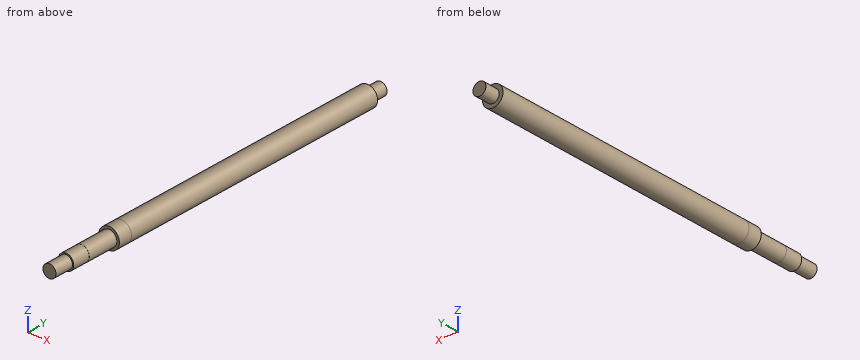
Autodesk Inventor part; units mm, degrees
ref_plane "YZ Plane" through (0, 0, 0) normal (1, 0, 0) x (0, 1, 0)
ref_plane "XZ Plane" through (0, 0, 0) normal (0, 1, 0) x (-1, 0, 0)
ref_plane "XY Plane" through (0, 0, 0) normal (0, 0, 1) x (1, 0, 0)
sketch "Sketch1" plane through (0, 0, 0) normal (0, 1, 0) x (-1, 0, 0)
  circle A0 centre (0, 0) radius 8
  dimension "d0" = 16
extrude "Extrusion1" add sketch "Sketch1" along normal blind 300
sketch "Sketch2" plane through (0, 0, 0) normal (0, -1, 0) x (1, 0, 0)
  circle A0 centre (0, 0) radius 8
extrude "Extrusion2" cut sketch "Sketch2" against normal blind 50
sketch "Sketch3" plane through (0, 50, 0) normal (0, -1, 0) x (1, 0, 0)
  circle A0 centre (0, 0) radius 8
extrude "Extrusion3" add sketch "Sketch3" along normal blind 50
sketch "Sketch4" plane through (0, 0, 0) normal (0, -1, 0) x (1, 0, 0)
  circle A0 centre (0, 0) radius 8
  circle A1 centre (0, 0) radius 6
  dimension "d7" = 12
extrude "Extrusion4" cut sketch "Sketch4" against normal blind 14
thread "Thread1"
sketch "Sketch6" plane through (0, 14, 0) normal (0, -1, 0) x (1, 0, 0)
  circle A0 centre (0, 0) radius 8
  circle A1 centre (0, 0) radius 6.05
  dimension "d13" = 12.1
extrude "Extrusion5" cut sketch "Sketch6" against normal blind 25
sketch "Sketch7" plane through (0, 0, 0) normal (0, -1, 0) x (1, 0, 0)
  circle A0 centre (0, 0) radius 6
  circle A1 centre (0, 0) radius 5
  dimension "d16" = 10
extrude "Extrusion6" add sketch "Sketch7" along normal blind 15 contours A1
sketch "Sketch8" plane through (0, 300, 0) normal (0, 1, 0) x (1, 0, 0)
  circle A0 centre (0, 0) radius 8
extrude "Extrusion7" cut sketch "Sketch8" against normal blind 27.101
sketch "Sketch9" plane through (0, 272.899, 0) normal (0, 1, 0) x (1, 0, 0)
  circle A0 centre (0, 0) radius 8
  circle A1 centre (0, 0) radius 5
  dimension "d21" = 10
extrude "Extrusion8" add sketch "Sketch9" along normal blind 12 contours A1
properties part number "1605_300mm"
Verification items for the finished model (mm, model axes). Coordinates: 2 decimals unless noted, no trailing zeros. Loops run counter-clockwise (first coordinate to the right, second up) from the corner with the lowest first, then second, coordinate; pieces in that order, holes last. Notation, with made-up numbers: (-24.75, -18) -> (-19.75, -18) arc R32 ccw to (-19.75, 8) -> close; hole circle Ø8 at (0.5, -29.75). An arc over 180 degrees is marked (long way). Answer as a JSON object with one key per item and string values. Group by question number.
Item 1: Sectioned sample at C-C on y = 123. Record the boundary of the cut face in (x, z), plus the area to 3 significant figures.
Item 2: Sectioned sample at B-B on x = 0. Record the boundary of the cut face in (y, z).
Item 3: Sectioned sample at A-A on z = 0. Record the boundary of the cut face in (x, y), plus the area to 3 significant figures.
Item 4: Scan lines: probe 1 along X at (y, z) = (218.5, -0.5); probe 2 along Y at (x, z) = (-3.25, -6.5); probe 3 along Z at (x, y) = (-5.25, 91.5). Record each from-to range of solid material in increasing order.
Item 5: Depth check by flat-ended pin: pin 1 (3 mm diameter, centred on y = 42.5, z = 5, fed in from +X); pin 2 (5 mm diameter, centred on x = 6, y = 151, fed in from -Z); pin 3 (8 mm diameter, centred on x = 5, z = 5, fed in from -Y); pin 4 (3 mm diameter, centred on y = 214, z = -4.5, fed in from -X). Enter the tip coordinate at first touch or a pass-through.
Evaluation:
{
 "1": {"outline": "circle Ø16 at (0, 0)", "area": "201 mm²"},
 "2": {"outline": "(-15, -5) -> (0, -5) -> (0, -6) -> (14, -6) -> (14, -6.05) -> (39, -6.05) -> (39, -8) -> (272.9, -8) -> (272.9, -5) -> (284.9, -5) -> (284.9, 5) -> (272.9, 5) -> (272.9, 8) -> (39, 8) -> (39, 6.05) -> (14, 6.05) -> (14, 6) -> (0, 6) -> (0, 5) -> (-15, 5) -> close"},
 "3": {"outline": "(-8, 39) -> (-6.05, 39) -> (-6.05, 14) -> (-6, 14) -> (-6, 0) -> (-5, 0) -> (-5, -15) -> (5, -15) -> (5, 0) -> (6, 0) -> (6, 14) -> (6.05, 14) -> (6.05, 39) -> (8, 39) -> (8, 272.9) -> (5, 272.9) -> (5, 284.9) -> (-5, 284.9) -> (-5, 272.9) -> (-8, 272.9) -> close", "area": "4,480 mm²"},
 "4": {"probe 1": "x = -7.98 to 7.98", "probe 2": "y = 39 to 272.9", "probe 3": "z = -6.04 to 6.04"},
 "5": {"pin 1": "stops at x = 7.19", "pin 2": "stops at z = -7.19", "pin 3": "stops at y = -15", "pin 4": "stops at x = -7.42"}
}
